from build123d import *

# Parameters (mm, degrees)
BOSS_EXTRUDE1_DEPTH = 10


with BuildPart() as part:
    # Sketch1 → Boss-Extrude1 (new body)
    with BuildSketch(Plane(origin=(0, 0, 0), x_dir=(1, 0, 0), z_dir=(0, 1, 0))):
        with BuildLine():
            Line((-20, 0), (-15.985928344, 0))
            ThreePointArc((-15.985928344, 0), (-15.954496575, 1.001970088), (-15.860324871, 2))
            Line((-15.860324871, 2), (-19.202832359, 2))
            Line((-19.202832359, 2), (-20, 2))
            Line((-20, 2), (-20, 0))
        make_face()
        with BuildLine():
            Line((-15.985928344, 0), (-12.5, 0))
            ThreePointArc((-12.5, 0), (0, 12.5), (12.5, 0))
            Line((12.5, 0), (15.985928344, 0))
            ThreePointArc((15.985928344, 0), (15.954496575, 1.001970088), (15.860324871, 2))
            ThreePointArc((15.860324871, 2), (0, 15.985928344), (-15.860324871, 2))
            ThreePointArc((-15.860324871, 2), (-15.954496575, 1.001970088), (-15.985928344, 0))
        make_face()
        with BuildLine():
            ThreePointArc((15.860324871, 2), (15.954496575, 1.001970088), (15.985928344, 0))
            Line((15.985928344, 0), (20, 0))
            Line((20, 0), (20, 2))
            Line((20, 2), (19.202832359, 2))
            Line((19.202832359, 2), (15.860324871, 2))
        make_face()
    extrude(amount=BOSS_EXTRUDE1_DEPTH)


solid = part.part
Verification items for the finished model (mm, model axes). A direction names the side the tool comes from. Coordinates: 2 decimals unless noted, no trailing zeros. Order: outer loops, then holes, each group sorted by start corner. A loop starts at its lowest first (then second) coordinate and runs counter-clockwise, first axis right, second up. Notation, with made-up numbers: M -37,25.5 L -28,25.5 A22 cw -28,62.5 Z; hole C -17,53.5 d11. An arc over 180 degrees is marked long. One line per item, written item: value. Start each with the question number.
Item 1: Sectioned sample at C-C (x = 0). Enter the section's corners in (y, z).
Item 2: Sectioned sample at B-B (x = -17). Enter the section's corners in (y, z), then the cut area to 3 significant figures.
Item 3: Sectioned sample at A-A (y = 9). Enter the section's corners in (x, z), then the cut area to 3 significant figures.
Item 4: Access from +Z, -Z, +X, -X, +Y, -Y to the whole of each face (thin tool, end or side, straight path). Record for faces 1 (the flat face through (-20, 5, -1)), 2 (the flat face through (18, 5, -2)).
Item 5: Gauge pin test, flat ends, axial feed: pin 1 (4.5 mm diameter, centred on x = -19, y = 5, fed in from -Z); pin 2 (6 mm diameter, centred on y = 8, z = -12.5, fed in from -X); pin 3 (6 mm diameter, centred on x = -12.5, y = 7.5, fed in from -Z). Record the tip position at first contact, or that the pin passes through.
Item 6: Mould release check, pull along X, two halves, no side actions. Record for faces 3 (the cylindrical face through (0.323, 4.93, -15.983)), 4 (the cylindrical face through (-0.275, 4.93, -12.497)), 5 (the flat face through (-18, 5, -2)), 6 (the flat face through (20, 5, -1)): released by +X, released by -X, zero draft, split by the parting line, or undercut.
Item 7: Scan lines: probe 1 along Z at (x, y) = (16.5, 1.5); probe 2 along X at (y, z) = (7, -8.75); probe 3 along X at (y, z) = (4.5, -1.25). Record each from-to range of solid material in increasing order.
Conclusion:
1. outline: M 0,-15.99 L 10,-15.99 L 10,-12.5 L 0,-12.5 Z
2. outline: M 0,-2 L 10,-2 L 10,0 L 0,0 Z
2. area: 20.0 mm^2
3. outline: M -20,-2 L -15.86,-2 A15.99 ccw 15.86,-2 L 20,-2 L 20,0 L 12.5,0 A12.5 cw -12.5,0 L -20,0 Z
3. area: 172 mm^2
4. face 1: +Z, -Z, -X, +Y, -Y
4. face 2: -Z, +X, +Y, -Y
5. pin 1: stops at z = -2
5. pin 2: stops at x = -12.86
5. pin 3: stops at z = -12.86
6. face 3: split by the parting line
6. face 4: undercut
6. face 5: zero draft
6. face 6: released by +X
7. probe 1: z = -2 to 0
7. probe 2: x = -13.38 to -8.93, 8.93 to 13.38
7. probe 3: x = -20 to -12.44, 12.44 to 20
